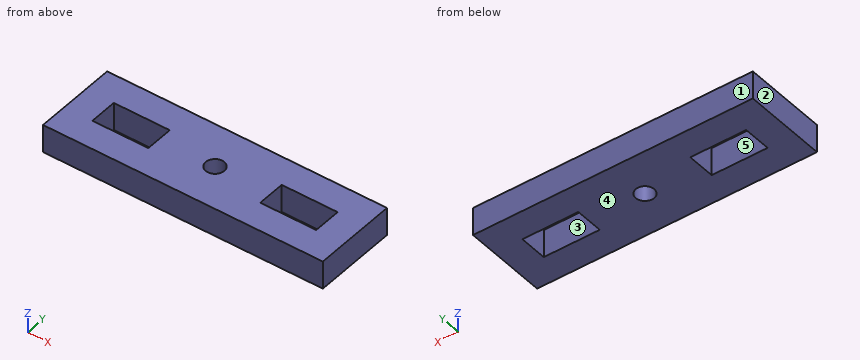
```python
from build123d import *

# Parameters (mm, degrees)
SKETCH1_W           = 63.5
SKETCH1_H           = 19.05
BOSS_EXTRUDE1_DEPTH = 6.35
SKETCH2_R           = 2.0955
SKETCH2_W           = 12.7
SKETCH2_H           = 6.35
CUT_EXTRUDE1_DEPTH  = 6.35


with BuildPart() as part:
    # Sketch1 → Boss-Extrude1 (new body)
    with BuildSketch(Plane.XY):
        Rectangle(SKETCH1_W, SKETCH1_H)
    extrude(amount=BOSS_EXTRUDE1_DEPTH)

    # Sketch2 → Cut-Extrude1 (cut)
    with BuildSketch(Plane.XY.offset(6.35)):
        Circle(SKETCH2_R)
        with Locations((-19.05, 0)):
            Rectangle(SKETCH2_W, SKETCH2_H)
        with Locations((19.05, 0)):
            Rectangle(SKETCH2_W, SKETCH2_H)
    extrude(amount=-CUT_EXTRUDE1_DEPTH, mode=Mode.SUBTRACT)


solid = part.part
```
Verification items for the finished model (mm, model axes). Face numbers are marked on the shaded views. A direction names the side the tool comes from. Round coordinates to 2 decimals unless told otherwise and drop trailing zeros. Order: outer loops, then holes, each group sorted by start corner. A loop starts at its lowest first (then second) coordinate and runs counter-clockwise, first axis right, second up. Notation, with made-up numbers: (43.25, 16) -> (65.25, 16) arc R11 cw to (65.25, 23) -> close; hole circle Ø11 at (43, 10.25). An arc over 180 degrees is marked (long way). Put each result on its own line as item: value. Start each with the question number.
(1) Section check A-A (x = 20). Enter the section's corners in (y, z) (3 decimals).
(2) Section check C-C (z = 2). State how many separate pieces and enclosed holes the cut face has, then the cut area to 3 significant figures.
(3) Material ranges on line 1 along Y through (x, z) = (0, 3.5) (1 decimal); line 2 along X through (y, z) = (-1.5, 3); line 3 along Y through (x, z) = (18, 3.5) (3 decimals), recorded low to high.
(4) Draft check along X on the marked faces 1, 2 and 3. Enter one of: +X half, -X half, draft (parallel to the pull), parting line (faces both ways), or undercut.
(5) Tool access check on the marked faces 4 and 5. Record the directions out of +Z, -Z, +X, -X, +Y, -Y that give a thin tool (end or side, any length) a straight path to the whole face; none if there is none.
(6) Section check B-B (y = 0). Enter the section's corners in (x, z).
Completed:
1. outline: (-9.525, 0) -> (-3.175, 0) -> (-3.175, 6.35) -> (-9.525, 6.35) -> close; (3.175, 0) -> (9.525, 0) -> (9.525, 6.35) -> (3.175, 6.35) -> close
2. separate pieces: 1
2. enclosed holes: 3
2. area: 1,030 mm2
3. line 1: y = -9.5 to -2.1, 2.1 to 9.5
3. line 2: x = -31.75 to -25.4, -12.7 to -1.46, 1.46 to 12.7, 25.4 to 31.75
3. line 3: y = -9.525 to -3.175, 3.175 to 9.525
4. face 1: draft
4. face 2: -X half
4. face 3: undercut
5. face 4: -Z, +X, -X, +Y, -Y
5. face 5: +Z, -Z
6. outline: (-31.75, 0) -> (-25.4, 0) -> (-25.4, 6.35) -> (-31.75, 6.35) -> close; (-12.7, 0) -> (-2.1, 0) -> (-2.1, 6.35) -> (-12.7, 6.35) -> close; (2.1, 0) -> (12.7, 0) -> (12.7, 6.35) -> (2.1, 6.35) -> close; (25.4, 0) -> (31.75, 0) -> (31.75, 6.35) -> (25.4, 6.35) -> close
